from build123d import *

# Parameters (mm, degrees)
SKETCH_3_R          = 2.15
CUT_EXTRUDE_2_DEPTH = 10


with BuildPart() as part:
    # 草图1 → 旋转1 (revolve)
    with BuildSketch(Plane(origin=(0, 0, 0), x_dir=(1, 0, 0), z_dir=(0, 1, 0))):
        Polygon((24.1, 0), (38.1, 0), (38.1, 6.1), (24.1, 6.1), (24.1, 8.05), (22.1, 8.05), (22.1, -1.95), (24.1, -1.95), align=None)
    revolve(axis=Axis((0, 0, 0), (0, 0, -1)))

    # 草图3 → 切除-拉伸2 (cut)
    with BuildSketch(Plane(origin=(0, 0, -6.1), x_dir=(-1, 0, 0), z_dir=(0, 0, -1))):
        with Locations((-32.1, 0)):
            Circle(SKETCH_3_R)
        with Locations((-16.05, 27.799415461)):
            Circle(SKETCH_3_R)
        with Locations((16.05, 27.799415461)):
            Circle(SKETCH_3_R)
        with Locations((32.1, 0)):
            Circle(SKETCH_3_R)
        with Locations((16.05, -27.799415461)):
            Circle(SKETCH_3_R)
        with Locations((-16.05, -27.799415461)):
            Circle(SKETCH_3_R)
    extrude(amount=-CUT_EXTRUDE_2_DEPTH, mode=Mode.SUBTRACT)


solid = part.part
The listing builds one solid part. Answer for the finished solid, in the listing's coordinates (mm). A direction names the side the tool comes from. Give positions to 0.01 mm unless a question says otherwise; leave off trailing zeros. Loops run counter-clockwise (first coordinate to the right, second up) from the corner with the lowest first, then second, coordinate; pieces in that order, holes last.
Item 1: Determine the mould class of faces 3 (the flat face through (1, 25, 0)), 4 (the cylindrical face through (30.05, 0.65, -3.09)), 5 (the cylindrical face through (-17.76, -16.29, 0.96)) for opening direction X: +X half, -X half, draft (parallel to the pull), parting line (faces both ways), or undercut.
Derived:
face 3: draft
face 4: undercut
face 5: parting line
Item 2: A cutting plane is placed at C-C (x = -16.05). Give the vertices of the cut face in (y, z), then the cut area to 3 significant figures.
Derived:
outline: (-34.55, -6.1) - (-29.95, -6.1) - (-29.95, 0) - (-34.55, 0) - close; (-25.65, -6.1) - (-17.98, -6.1) - (-17.98, -8.05) - (-15.19, -8.05) - (-15.19, 1.95) - (-17.98, 1.95) - (-17.98, 0) - (-25.65, 0) - close; (15.19, -8.05) - (17.98, -8.05) - (17.98, -6.1) - (25.65, -6.1) - (25.65, 0) - (17.98, 0) - (17.98, 1.95) - (15.19, 1.95) - close; (29.95, -6.1) - (34.55, -6.1) - (34.55, 0) - (29.95, 0) - close
area: 205 mm2
Item 3: A cutting plane is placed at D-D (x = -32.1). Give the vertices of the cut face in (y, z).
Derived:
outline: (-20.52, -6.1) - (-2.15, -6.1) - (-2.15, 0) - (-20.52, 0) - close; (2.15, -6.1) - (20.52, -6.1) - (20.52, 0) - (2.15, 0) - close
Item 4: Each of these flat-tipped pins is pushed along its axis until it touches: pin 1 Ø4 at (x, y) = (27, 21) entering from +Z; pin 2 Ø1.5 at (x, z) = (-2, -1.5) entering from -Y; pin 3 Ø2 at (y, z) = (-2, -6) entering from +X. Where does it stop, or does it pass through?
Derived:
pin 1: stops at z = 0
pin 2: stops at y = -38.08
pin 3: stops at x = 38.09
Item 5: A cutting plane is placed at A-A (x = 0). Give the vertices of the cut face in (y, z), then the cut area to 3 significant figures.
Derived:
outline: (-38.1, -6.1) - (-24.1, -6.1) - (-24.1, -8.05) - (-22.1, -8.05) - (-22.1, 1.95) - (-24.1, 1.95) - (-24.1, 0) - (-38.1, 0) - close; (22.1, -8.05) - (24.1, -8.05) - (24.1, -6.1) - (38.1, -6.1) - (38.1, 0) - (24.1, 0) - (24.1, 1.95) - (22.1, 1.95) - close
area: 211 mm2
Item 6: Find the intervals of material crossed by line 1 along X through (y, z) = (-29.5, -6); line 2 along X through (y, z) = (29, -1.5); line 3 along Y through (x, z) = (-15, -0.5), in increasing order.
Derived:
line 1: x = -24.11 to -17.37, -14.73 to 14.73, 17.37 to 24.11
line 2: x = -24.71 to -17.83, -14.27 to 14.27, 17.83 to 24.71
line 3: y = -35.02 to -29.68, -25.92 to -16.23, 16.23 to 25.92, 29.68 to 35.02
Item 7: A cutting plane is placed at B-B (y = -7). Give the vertices of the cut face in (x, z), then the cut area to 3 significant figures.
Derived:
outline: (-37.45, -6.1) - (-23.06, -6.1) - (-23.06, -8.05) - (-20.96, -8.05) - (-20.96, 1.95) - (-23.06, 1.95) - (-23.06, 0) - (-37.45, 0) - close; (20.96, -8.05) - (23.06, -8.05) - (23.06, -6.1) - (37.45, -6.1) - (37.45, 0) - (23.06, 0) - (23.06, 1.95) - (20.96, 1.95) - close
area: 218 mm2
Item 8: A tool of negligible diameter and unlimited length cuts with its end or side. For faces 1 (the flat face through (-1, 25, -6.1)), 2 (the cylindrical face through (-30.235, 23.183, -3.093)), from which of +Z, -Z, +X, -X, +Y, -Y can it reach the whole face along a straight path? Write none if from no direction.
Derived:
face 1: -Z
face 2: +Z, -Z
